from build123d import *

# Parameters (mm, degrees)
SKETCH1_W            = 193
SKETCH1_H            = 116.5
SKETCH1_R            = 1.75
SKETCH1_R_2          = 8
SKETCH1_W_2          = 2
SKETCH1_H_2          = 55
BOSS_EXTRUDE1_DEPTH  = 6
SKETCH3_W            = 10
SKETCH3_H            = 10
BOSS_EXTRUDE3_DEPTH  = 10
SKETCH5_W            = 2
SKETCH5_H            = 55
BOSS_EXTRUDE4_DEPTH  = 6
SKETCH6_W            = 181
SKETCH6_H            = 104.5
CUT_EXTRUDE1_DEPTH   = 4
SKETCH7_W            = 1.5
SKETCH7_H            = 55
BOSS_EXTRUDE5_DEPTH  = 44.75
SKETCH8_W            = 2
SKETCH8_H            = 55
CUT_EXTRUDE2_DEPTH   = 42.25
FILLET3_R            = 3
SKETCH12_W           = 55
SKETCH12_H           = 2
BOSS_EXTRUDE6_DEPTH  = 1.5
SKETCH14_W           = 3
SKETCH14_H           = 44.75
BOSS_EXTRUDE7_DEPTH  = 2
SKETCH15_W           = 3
SKETCH15_H           = 44.75
BOSS_EXTRUDE8_DEPTH  = 2
BOSS_EXTRUDE9_DEPTH  = 2
SKETCH18_W           = 20
SKETCH18_H           = 32.75
BOSS_EXTRUDE10_DEPTH = 2


with BuildPart() as part:
    # Sketch1 → Boss-Extrude1 (new body)
    with BuildSketch(Plane(origin=(0, 0, 0), x_dir=(1, 0, 0), z_dir=(0, 1, 0))):
        with Locations((22.87983871, -17.078434096)):
            Rectangle(SKETCH1_W, SKETCH1_H)
        with Locations(Location((-70.62016129, -72.328434096, 0), (0, 0, 270))):
            Circle(SKETCH1_R, mode=Mode.SUBTRACT)
        with Locations(Location((-70.62016129, 38.171565904, 0), (0, 0, 270))):
            Circle(SKETCH1_R, mode=Mode.SUBTRACT)
        with Locations(Location((116.37983871, -72.328434096, 0), (0, 0, 270))):
            Circle(SKETCH1_R, mode=Mode.SUBTRACT)
        with Locations(Location((116.37983871, 38.171565904, 0), (0, 0, 270))):
            Circle(SKETCH1_R, mode=Mode.SUBTRACT)
        with Locations(Location((82.450678359, -17.078434096, 0), (0, 0, 270))):
            Circle(SKETCH1_R_2, mode=Mode.SUBTRACT)
        with Locations((-47.331266899, -17.078434096)):
            Rectangle(SKETCH1_W_2, SKETCH1_H_2, mode=Mode.SUBTRACT)
    extrude(amount=BOSS_EXTRUDE1_DEPTH)

    # Sketch3 → Boss-Extrude3 (add)
    with BuildSketch(Plane.XZ):
        with Locations((-62.62016129, 64.328434096)):
            Rectangle(SKETCH3_W, SKETCH3_H)
        with Locations((-62.62016129, -30.171565904)):
            Rectangle(SKETCH3_W, SKETCH3_H)
        with Locations((108.37983871, -30.171565904)):
            Rectangle(SKETCH3_W, SKETCH3_H)
        with Locations((108.37983871, 64.328434096)):
            Rectangle(SKETCH3_W, SKETCH3_H)
    extrude(amount=BOSS_EXTRUDE3_DEPTH)

    # Sketch5 → Boss-Extrude4 (add)
    with BuildSketch(Plane.XZ):
        with Locations((-47.331266899, 17.078434096)):
            Rectangle(SKETCH5_W, SKETCH5_H)
    extrude(amount=-BOSS_EXTRUDE4_DEPTH)

    # Sketch6 → Cut-Extrude1 (cut)
    with BuildSketch(Plane.XZ.offset(10)):
        with Locations((22.87983871, 17.078434096)):
            Rectangle(SKETCH6_W, SKETCH6_H)
    extrude(amount=-CUT_EXTRUDE1_DEPTH, mode=Mode.SUBTRACT)

    # Sketch7 → Boss-Extrude5 (add)
    with BuildSketch(Plane.XZ):
        with Locations((-61.87016129, 17.078434096)):
            Rectangle(SKETCH7_W, SKETCH7_H)
    extrude(amount=BOSS_EXTRUDE5_DEPTH)

    # Sketch8 → Cut-Extrude2 (cut)
    with BuildSketch(Plane.XZ):
        with Locations((-60.12016129, 17.078434096)):
            Rectangle(SKETCH8_W, SKETCH8_H)
    extrude(amount=-CUT_EXTRUDE2_DEPTH, mode=Mode.SUBTRACT)

    # Fillet3
    fillet3_edges = [part.edges().sort_by_distance(p)[0] for p in [
        (-67.62016129, -6, 64.328434096),
        (-67.62016129, -6, -30.171565904),
        (-62.62016129, -6, -35.171565904),
        (108.37983871, -6, -35.171565904),
        (-62.62016129, -6, 69.328434096),
        (108.37983871, -6, 69.328434096),
        (113.37983871, -6, -30.171565904),
        (113.37983871, -6, 64.328434096),
        (-62.62016129, -6, 59.328434096),
        (-57.62016129, -6, 64.328434096),
        (103.37983871, -6, 64.328434096),
        (108.37983871, -6, 59.328434096),
        (108.37983871, -6, -25.171565904),
        (103.37983871, -6, -30.171565904),
        (-57.62016129, -6, -30.171565904),
        (-62.62016129, -6, -25.171565904),
    ]]
    fillet(fillet3_edges, radius=FILLET3_R)

    # Sketch12 → Boss-Extrude6 (add)
    with BuildSketch(Plane(origin=(-61.12016129, 0, 0), x_dir=(0, 0, -1), z_dir=(1, 0, 0))):
        with Locations((-17.078434096, -43.75)):
            Rectangle(SKETCH12_W, SKETCH12_H)
    extrude(amount=BOSS_EXTRUDE6_DEPTH)

    # Sketch14 → Boss-Extrude7 (add)
    with BuildSketch(Plane(origin=(0, 0, -10.421565904), x_dir=(-1, 0, 0), z_dir=(0, 0, -1))):
        with Locations((61.12016129, -22.375)):
            Rectangle(SKETCH14_W, SKETCH14_H)
    extrude(amount=BOSS_EXTRUDE7_DEPTH)

    # Sketch15 → Boss-Extrude8 (add)
    with BuildSketch(Plane.XY.offset(44.578434096)):
        with Locations((-61.12016129, -22.375)):
            Rectangle(SKETCH15_W, SKETCH15_H)
    extrude(amount=BOSS_EXTRUDE8_DEPTH)

    # Sketch16 → Boss-Extrude9 (add)
    with BuildSketch(Plane.ZY.offset(62.62016129)):
        Polygon((-10.421565904, 0), (-10.421565904, -42.75), (46.578434096, -42.75), (46.578434096, -44.75), (-12.421565904, -44.75), (-12.421565904, 0), align=None)
    extrude(amount=BOSS_EXTRUDE9_DEPTH)

    # Sketch18 → Boss-Extrude10 (add)
    with BuildSketch(Plane(origin=(-59.62016129, 0, 0), x_dir=(0, 0, -1), z_dir=(1, 0, 0))):
        with Locations((-36.578434096, -16.375)):
            Rectangle(SKETCH18_W, SKETCH18_H)
        with Locations((2.421565904, -16.375)):
            Rectangle(SKETCH18_W, SKETCH18_H)
    extrude(amount=BOSS_EXTRUDE10_DEPTH)


solid = part.part
Could you check a few things on this model? Use its own coordinates, in mm. A direction names the side the tool comes from. Give positions to 0.01 mm unless a question says otherwise; leave off trailing zeros. Order: outer loops, then holes, each group sorted by start corner. A loop starts at its lowest first (then second) coordinate and runs counter-clockwise, first axis right, second up. Notation, with made-up numbers: (-11.75, 71) - (34.25, 71) arc R27 ccw to (34.25, 87) - close; hole circle Ø3 at (-26, -32). An arc over 180 degrees is marked (long way). Return JSON: item names as keys, results as strings. Group by question number.
Q1. Suppose I cut it at B-B, the plane y = -39. Please give me the cut outline in (x, z).
Q2. Which directions (+Z, -Z, +X, -X, +Y, -Y) give clear straight access to the entire face, cutting with the end or side of a thin tool? Please do faces 1 (the face through (117.855, 2.958, -37.231)), 2 (the face through (22, 3, 75.328)), 3 (the face through (-59.12, 3, 17)), 4 (the face through (-57.62, -16, -2)), 5 (the face through (-61, -23, -12.422)).
Q3. Thinking about a two-plate mould opening in X: for faces 6 (the face through (118.115, 2.958, 72.101)), 7 (the face through (119.38, 3, 18)), 8 (the face through (-63, -6, -30)), which applies, pulls with the +X half, pulls with the -X half, needs draft (parallel to the pull), parting line crosses it, or undercut?
Q4. Please list where these lines run through material, in increasing order: line 1 along Z through (x, y) = (108, -1); line 2 along X through (y, z) = (-15, 44); line 3 along X through (y, z) = (4.5, 23). Write a range as [from, to].
Q5. Suppose I cut it at C-C, the plane z = 12.5. Please give me the cut outline in (x, y).
Q6. Suppose I cut it at A-A, the plane z = -7. Please give me the cut outline in (x, y), and give its area (3 significant figures).
Q7. Suppose I cut it at D-D, the plane x = 4. Please give me the cut outline in (y, z).
Q8. Will these pins go through, and if not, where does the flat tip stop? pin 1 Ø10 at (x, z) = (84.5, 54) entering from -Y; pin 2 Ø1.5 at (x, y) = (109, -1.5) entering from +Z; pin 3 Ø9.5 at (y, z) = (-37.5, 19) entering from +X.
Resolved:
{
 "1": {"outline": "(-64.62, -12.42) - (-59.62, -12.42) - (-59.62, -10.42) - (-61.12, -10.42) - (-61.12, 44.58) - (-59.62, 44.58) - (-59.62, 46.58) - (-62.62, 46.58) - (-62.62, -10.42) - (-64.62, -10.42) - close"},
 "2": {"face 1": "+Y, -Y", "face 2": "+Z, +X, -X, +Y, -Y", "face 3": "+Y", "face 4": "+Z, -Z, +X, -Y", "face 5": "+X, -X, -Y"},
 "3": {"face 6": "undercut", "face 7": "pulls with the +X half", "face 8": "needs draft"},
 "4": {"line 1": "z = [-35.17, -25.17], [59.33, 69.33]", "line 2": "x = [-62.62, -61.12], [-59.62, -57.62]", "line 3": "x = [-73.62, -61.12], [-59.12, 77.07], [87.83, 119.38]"},
 "5": {"outline": "(-73.62, 0) - (-62.62, 0) - (-62.62, -42.75) - (-64.62, -42.75) - (-64.62, -44.75) - (-59.62, -44.75) - (-59.62, -42.75) - (-61.12, -42.75) - (-61.12, 6) - (-73.62, 6) - close; (-59.12, 0) - (75.89, 0) - (75.89, 6) - (-59.12, 6) - close; (89.01, 0) - (119.38, 0) - (119.38, 6) - (89.01, 6) - close"},
 "6": {"outline": "(-73.62, 0) - (-62.62, 0) - (-62.62, -42.75) - (-64.62, -42.75) - (-64.62, -44.75) - (-59.62, -44.75) - (-59.62, -42.75) - (-61.12, -42.75) - (-61.12, 6) - (-73.62, 6) - close; (-59.62, -32.75) - (-57.62, -32.75) - (-57.62, 0) - (119.38, 0) - (119.38, 6) - (-59.12, 6) - (-59.12, 0) - (-59.62, 0) - close", "area": "1,290 mm2"},
 "7": {"outline": "(0, -41.17) - (6, -41.17) - (6, 75.33) - (0, 75.33) - close"},
 "8": {"pin 1": "stops at y = 0", "pin 2": "stops at z = 69.33", "pin 3": "stops at x = -61.12"}
}
